CAD build for the part. Positions are in the model's coordinates, mm. A direction names the side the tool comes from. Round coordinates to 2 decimals unless told otherwise and drop trailing zeros. Loops run counter-clockwise (first coordinate to the right, second up) from the corner with the lowest first, then second, coordinate; pieces in that order, holes last. Notation, with made-up numbers: M -13.5,42.5 L 43.5,42.5 A24 cw 43.5,58.5 Z; hole C 12,-27 d10. An arc over 180 degrees is marked long. Use a Markdown table: item, result. Add a question column.
(1) Wall check: L1, parallel to X at y = 7.5, z = 5.75; L2, parallel to Y at x = -25.5, z = 4.75; L3, parallel to X at y = 114, z = 5.75. Give the ranges that are in metal, low to high.
(2) Band-saw the part on C-C, the plane x = 0. Write the cut outline in (y, z), and give its area (3 significant figures).
(3) Flat gauge pins, fed straight in: P1, Ø3, axis at x = 39, z = 0.5, coming from the -Y side; P2, Ø1.9, axis at y = 107, z = 2.5, coming from the +X side; P3, Ø3, axis at x = -26.5, z = 3.5, coming from the +Y side. Where does each tip first touch, or does it go through?
(4) Two-plate mould, pull along Y, no slides. Class faces 1 (the face through (-107.557, 1.625, 3.131)), 2 (the face through (-120.94, -92.73, 3.13)), 3 (the face through (-0.53, 36.89, 3.13)), 4 (the face through (32, 2, 0)): released by +Y, released by -Y, zero draft, split by the parting line, or undercut.
(5) Which spindle directions (+Z, -Z, +X, -X, +Y, -Y) get a long thin tool onto all of the face, cutting with end or side? Do faces 5 (the face through (32, 2, 6.35)), 6 (the face through (-0.385, -30.605, 3.131)). Say none if no direction does.
(6) Band-saw the part on A-A, the plane y = 0. Write the cut outline in (x, z), and give its area (3 significant figures).
(7) Band-saw the part on B-B, the plane z = 1. Write the cut outline in (x, y), and give its area (3 significant figures).
(8) Band-saw the part on D-D, the plane y = 82.5. Write the cut outline in (x, z), and give its area (3 significant figures).
from build123d import *

# Parameters (mm, degrees)
F0_R     = 152.4
F0_R_2   = 12.7
F1_DEPTH = 6.35


with BuildPart() as f1:
    # F0 (on Top) → F1 (new body)
    with BuildSketch(Plane.XY):
        Circle(F0_R)
        with BuildLine():
            ThreePointArc((31.594744, -19.05), (0, -36.8935), (-31.594744, -19.05))
            Line((-31.594744, -19.05), (-23.955917, -19.05))
            ThreePointArc((-23.955917, -19.05), (0, -30.607), (23.955917, -19.05))
            Line((23.955917, -19.05), (31.594744, -19.05))
        make_face(mode=Mode.SUBTRACT)
        with BuildLine():
            ThreePointArc((-50.8, -116.813009), (-127.381, 0), (-50.8, 116.813009))
            Line((-50.8, 116.813009), (-50.8, 94.817982))
            ThreePointArc((-50.8, 94.817982), (-107.569, 0), (-50.8, -94.817982))
            Line((-50.8, -94.817982), (-50.8, -116.813009))
        make_face(mode=Mode.SUBTRACT)
        Circle(F0_R_2, mode=Mode.SUBTRACT)
        with BuildLine():
            Line((-23.955917, 19.05), (-31.594744, 19.05))
            ThreePointArc((-31.594744, 19.05), (0, 36.8935), (31.594744, 19.05))
            Line((31.594744, 19.05), (23.955917, 19.05))
            ThreePointArc((23.955917, 19.05), (0, 30.607), (-23.955917, 19.05))
        make_face(mode=Mode.SUBTRACT)
        with BuildLine():
            Line((50.8, 94.817982), (50.8, 116.813009))
            ThreePointArc((50.8, 116.813009), (127.381, 0), (50.8, -116.813009))
            Line((50.8, -116.813009), (50.8, -94.817982))
            ThreePointArc((50.8, -94.817982), (107.569, 0), (50.8, 94.817982))
        make_face(mode=Mode.SUBTRACT)
    extrude(amount=F1_DEPTH)


solid = f1.part
Return value:
| question | item | result |
|---|---|---|
| 1 | L1 | -152.22 to -127.16, -107.31 to -10.25, 10.25 to 107.31, 127.16 to 152.22 |
| 1 | L2 | -150.25 to -26.66, -19.05 to 19.05, 26.66 to 150.25 |
| 1 | L3 | -101.14 to -56.83, -50.8 to 50.8, 56.83 to 101.14 |
| 2 | outline | M -152.4,0 L -36.89,0 L -36.89,6.35 L -152.4,6.35 Z; M -30.61,0 L -12.7,0 L -12.7,6.35 L -30.61,6.35 Z; M 12.7,0 L 30.61,0 L 30.61,6.35 L 12.7,6.35 Z; M 36.89,0 L 152.4,0 L 152.4,6.35 L 36.89,6.35 Z |
| 2 | area | 1,690 mm^2 |
| 3 | P1 | y = -147.71 |
| 3 | P2 | x = 109.45 |
| 3 | P3 | y = 150.34 |
| 4 | face 1 | undercut |
| 4 | face 2 | split by the parting line |
| 4 | face 3 | undercut |
| 4 | face 4 | zero draft |
| 5 | face 5 | +Z, +X, -X, +Y, -Y |
| 5 | face 6 | +Z, -Z |
| 6 | outline | M -152.4,0 L -127.38,0 L -127.38,6.35 L -152.4,6.35 Z; M -107.57,0 L -12.7,0 L -12.7,6.35 L -107.57,6.35 Z; M 12.7,0 L 107.57,0 L 107.57,6.35 L 12.7,6.35 Z; M 127.38,0 L 152.4,0 L 152.4,6.35 L 127.38,6.35 Z |
| 6 | area | 1,520 mm^2 |
| 7 | outline | C 0,0 d304.8; hole M -50.8,-116.81 L -50.8,-94.82 A107.57 cw -50.8,94.82 L -50.8,116.81 A127.38 ccw Z; hole M -31.59,-19.05 A36.89 ccw 31.59,-19.05 L 23.96,-19.05 A30.61 cw -23.96,-19.05 Z; hole M -31.59,19.05 L -23.96,19.05 A30.61 cw 23.96,19.05 L 31.59,19.05 A36.89 ccw Z; hole C 0,0 d25.4; hole M 50.8,-116.81 A127.38 ccw 50.8,116.81 L 50.8,94.82 A107.57 cw 50.8,-94.82 Z |
| 7 | area | 61,200 mm^2 |
| 8 | outline | M -128.14,0 L -97.05,0 L -97.05,6.35 L -128.14,6.35 Z; M -69.03,0 L 69.03,0 L 69.03,6.35 L -69.03,6.35 Z; M 97.05,0 L 128.14,0 L 128.14,6.35 L 97.05,6.35 Z |
| 8 | area | 1,270 mm^2 |
